The drawing under review shows one solid part. Ordinate dimensions are in mm from its lowest x, y, z. Coordinates: 2 decimals unless noted, no trailing zeros. Write each loop counter-clockwise with the first axis right and the second up, starting at its lowest first coordinate (ties: lowest second). Pieces come first, ordered by that corner, then holes.
Q1. Mouldability with a two-part tool opening along Y and no side actions: class the marked faces 1, 2, 3 and 4 as pulls with the +Y half, pulls with the -Y half, needs draft (parallel to the pull), parting line crosses it, or undercut.
Q2. Take a section at A-A (z = 34). Give the boundary of the cut face in (x, y).
Q3. Insertion check: pin 1 (4 mm diameter, centred on x = 29.5, z = 36.5, fed in from -Y). The pin has a flat end and moves straight along its axis. Give the tip position at first contact, or say it passes through.
Q4. Take a section at C-C (y = 17.5). Give the boundary of the cut face in (x, z).
Q5. For probe 1 along Y at (x, z) = (20, 14); probe 2 along Y at (x, z) = (4, 21); probe 3 along X at (y, z) = (38, 18.5), list the stretches that pass through material, from the lowest coordinate up.
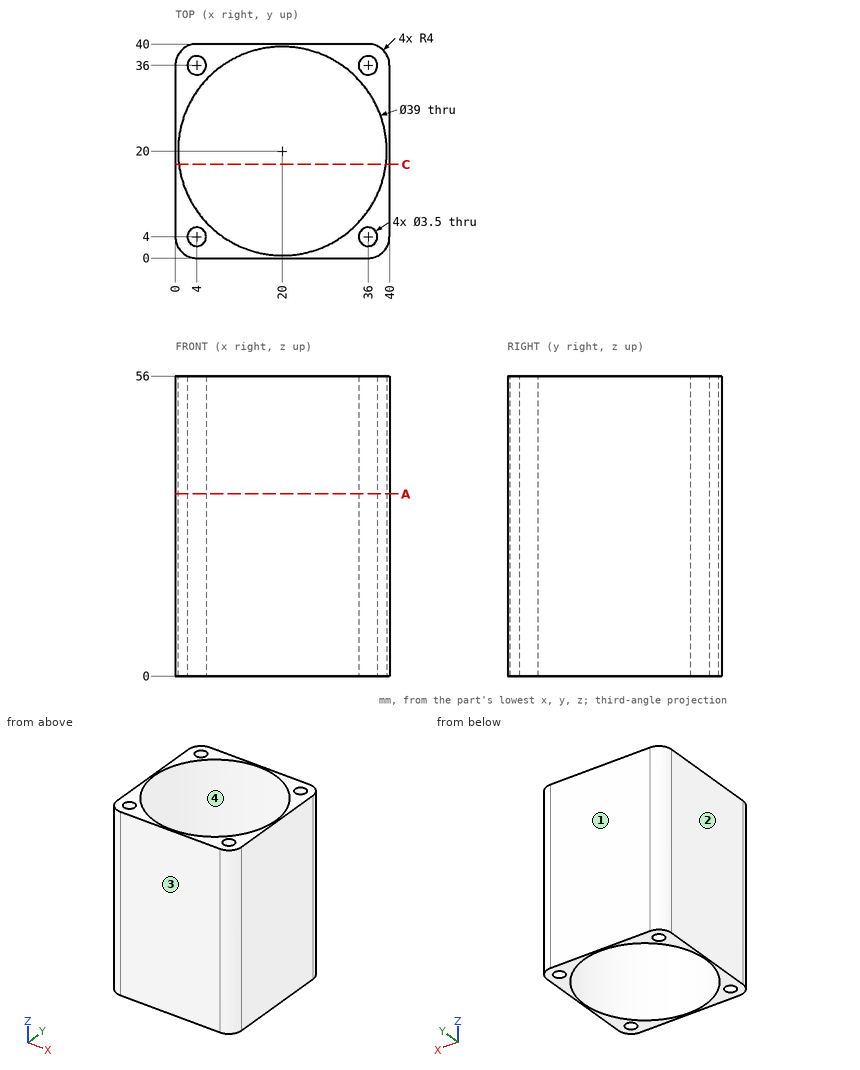
Response:
1. face 1: pulls with the +Y half
1. face 2: needs draft
1. face 3: pulls with the -Y half
1. face 4: undercut
2. outline: (0, 4) arc R4 ccw to (4, 0) - (36, 0) arc R4 ccw to (40, 4) - (40, 36) arc R4 ccw to (36, 40) - (4, 40) arc R4 ccw to (0, 36) - close; hole circle Ø39 at (20, 20); hole circle Ø3.5 at (4, 4); hole circle Ø3.5 at (4, 36); hole circle Ø3.5 at (36, 4); hole circle Ø3.5 at (36, 36)
3. pin 1: stops at y = 0
4. outline: (0, 0) - (0.66, 0) - (0.66, 56) - (0, 56) - close; (39.34, 0) - (40, 0) - (40, 56) - (39.34, 56) - close
5. probe 1: y = 0 to 0.5, 39.5 to 40
5. probe 2: y = 0 to 2.25, 5.75 to 8.85, 31.15 to 34.25, 37.75 to 40
5. probe 3: x = 0.54 to 12.5, 27.5 to 39.46
